CAD build for the part. Positions are in the model's coordinates, mm. Round coordinates to 2 decimals unless told otherwise and drop trailing zeros. Loops run counter-clockwise (first coordinate to the right, second up) from the corner with the lowest first, then second, coordinate; pieces in that order, holes last.
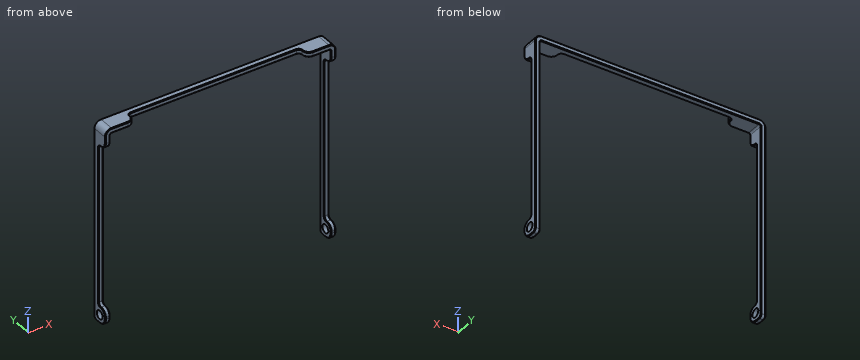
from build123d import *

# Parameters (mm, degrees)
EXTRUDE_1_DEPTH     = 5
FILLET_1_R          = 2
FILLET_2_R          = 0.5
FILLET_3_R          = 2.5
SKETCH_2_R          = 1.3
CUT_EXTRUDE_1_DEPTH = 100
SKETCH_3_W          = 52.2
SKETCH_3_H          = 6.2
CUT_EXTRUDE_2_DEPTH = 5
FILLET_5_R          = 1
SKETCH_4_W          = 49
SKETCH_4_H          = 8.82072143
CUT_EXTRUDE_3_DEPTH = 100
FILLET_6_R          = 1
FILLET_7_R          = 2
CHAMFER_1_SIZE      = 0.2


with BuildPart() as part:
    # 草图1 → 凸台-拉伸1 (new body)
    with BuildSketch(Plane(origin=(0, 0, 0), x_dir=(1, 0, 0), z_dir=(0, 1, 0))):
        Polygon((33.5, 29.25), (35, 29.25), (35, -30.75), (-35, -30.75), (-35, 29.25), (-33.5, 29.25), (-33.5, -29.25), (33.5, -29.25), align=None)
    extrude(amount=EXTRUDE_1_DEPTH)

    # 圆角1
    fillet_1_edges = [part.edges().sort_by_distance(p)[0] for p in [
        (35, 2.5, 30.75),
        (-35, 2.5, 30.75),
    ]]
    fillet(fillet_1_edges, radius=FILLET_1_R)

    # 圆角2
    fillet_2_edges = [part.edges().sort_by_distance(p)[0] for p in [
        (-33.5, 2.5, 29.25),
        (33.5, 2.5, 29.25),
    ]]
    fillet(fillet_2_edges, radius=FILLET_2_R)

    # 圆角3
    fillet_3_edges = [part.edges().sort_by_distance(p)[0] for p in [
        (-34.25, 0, -29.25),
        (34.25, 0, -29.25),
    ]]
    fillet(fillet_3_edges, radius=FILLET_3_R)

    # 草图2 → 切除-拉伸1 (cut)
    with BuildSketch(Plane.ZY.offset(35)):
        with Locations((-26.75, 2.5)):
            Circle(SKETCH_2_R)
    extrude(amount=-CUT_EXTRUDE_1_DEPTH, mode=Mode.SUBTRACT)

    # 草图3 → 切除-拉伸2 (cut)
    with BuildSketch(Plane.XY.offset(30.75)):
        Rectangle(SKETCH_3_W, SKETCH_3_H)
    extrude(amount=-CUT_EXTRUDE_2_DEPTH, mode=Mode.SUBTRACT)

    # 圆角5
    fillet_5_edges = [part.edges().sort_by_distance(p)[0] for p in [
        (-26.1, 3.1, 30),
        (26.1, 3.1, 30),
    ]]
    fillet(fillet_5_edges, radius=FILLET_5_R)

    # 草图4 → 切除-拉伸3 (cut)
    with BuildSketch(Plane.ZY.offset(35)):
        with Locations((0.25, -1.310360715)):
            Rectangle(SKETCH_4_W, SKETCH_4_H)
    extrude(amount=-CUT_EXTRUDE_3_DEPTH, mode=Mode.SUBTRACT)

    # 圆角6
    fillet_6_edges = [part.edges().sort_by_distance(p)[0] for p in [
        (34.25, 3.1, -24.25),
        (-34.25, 3.1, -24.25),
        (34.25, 3.1, 24.75),
        (-34.25, 3.1, 24.75),
        (-34.25, 5, -29.25),
        (34.25, 5, -29.25),
    ]]
    fillet(fillet_6_edges, radius=FILLET_6_R)

    # 圆角7
    fillet_7_edges = [part.edges().sort_by_distance(p)[0] for p in [
        (-34.25, 0, 24.75),
        (-34.25, 0, -24.25),
        (34.25, 0, -24.25),
        (34.25, 0, 24.75),
        (-26.1, 0, 30),
        (26.1, 0, 30),
    ]]
    fillet(fillet_7_edges, radius=FILLET_7_R)

    # 倒角1
    chamfer_1_edges = [part.edges().sort_by_distance(p)[0] for p in [
        (33.5, 5, 0.25),
        (-35, 5, 0.25),
        (-35, 2.05, -24.25),
        (-35, 3.1, 0.25),
        (-35, 3.25, -29.25),
        (-35, 4.707106781, -28.957106781),
        (-33.5, 3.25, -29.25),
        (-33.5, 3.1, 0.25),
        (-33.5, 2.05, -24.25),
        (-33.5, 4.707106781, -28.957106781),
        (33.5, 3.1, 0.25),
        (33.5, 2.05, 24.75),
        (33.5, 3.25, -29.25),
        (33.5, 4.707106781, -28.957106781),
        (35, 3.25, -29.25),
        (35, 3.1, 0.25),
        (35, 2.05, -24.25),
        (35, 4.707106781, -28.957106781),
        (33.5, 2.807106781, -23.957106781),
        (35, 2.807106781, -23.957106781),
        (33.5, 2.807106781, 24.457106781),
        (35, 2.807106781, 24.457106781),
        (-35, 2.807106781, 24.457106781),
        (-33.5, 2.807106781, 24.457106781),
        (-35, 2.807106781, -23.957106781),
        (-33.5, 2.807106781, -23.957106781),
        (35, 0, -26.5),
        (33.5, 2.05, -24.25),
        (33.5, 0, 27.75),
        (33.5, 0.585786438, 25.335786438),
        (33.5, 0.585786438, -24.835786438),
        (35, 2.05, 24.75),
        (35, 0.585786438, 25.335786438),
        (35, 0.585786438, -24.835786438),
        (-33.5, 0, -26.5),
        (-35, 2.05, 24.75),
        (-35, 0, 27.75),
        (-35, 0.585786438, 25.335786438),
        (-35, 0.585786438, -24.835786438),
        (-33.5, 2.05, 24.75),
        (-33.5, 0.585786438, 25.335786438),
        (-33.5, 0.585786438, -24.835786438),
        (-30.55, 0, 29.25),
        (26.1, 2.05, 30.75),
        (30.55, 0, 30.75),
        (26.685786438, 0.585786438, 30.75),
        (-26.685786438, 0.585786438, 30.75),
        (26.1, 2.05, 29.25),
        (26.685786438, 0.585786438, 29.25),
        (-26.685786438, 0.585786438, 29.25),
        (35, 0, 27.75),
        (35, 5, 0.25),
        (-30.55, 0, 30.75),
        (-34.414213562, 0, 30.164213562),
        (34.414213562, 0, 30.164213562),
        (0, 5, 30.75),
        (-34.414213562, 5, 30.164213562),
        (34.414213562, 5, 30.164213562),
        (30.55, 0, 29.25),
        (0, 5, 29.25),
        (-33.5, 0, 27.75),
        (-33.5, 5, 0.25),
        (33.353553391, 0, 29.103553391),
        (33.353553391, 5, 29.103553391),
        (-33.353553391, 0, 29.103553391),
        (-33.353553391, 5, 29.103553391),
        (33.5, 0, -26.5),
        (33.5, 0.732233047, -28.517766953),
        (-35, 0, -26.5),
        (35, 0.732233047, -28.517766953),
        (-35, 0.732233047, -28.517766953),
        (-33.5, 0.732233047, -28.517766953),
        (0, 3.1, 30.75),
        (0, 3.1, 29.25),
        (-26.1, 2.05, 30.75),
        (-26.1, 2.05, 29.25),
        (25.807106781, 2.807106781, 30.75),
        (25.807106781, 2.807106781, 29.25),
        (-25.807106781, 2.807106781, 30.75),
        (-25.807106781, 2.807106781, 29.25),
    ]]
    chamfer(chamfer_1_edges, length=CHAMFER_1_SIZE)


solid = part.part
Item 1: Flat gauge pins, fed straight in: P1, Ø2.5, axis at x = -3.5, y = 2, coming from the -Z side; P2, Ø0.9, axis at x = 34, z = -9.5, coming from the -Y side. Where does each tip first touch, or does it go through?
Verdict:
P1: stops at z = 29.3
P2: stops at y = 3.1
Item 2: Cut at C-C (x = 1.5). List the corners of the cut face in (y, z).
Verdict:
outline: (3.1, 29.45) - (3.3, 29.25) - (4.8, 29.25) - (5, 29.45) - (5, 30.55) - (4.8, 30.75) - (3.3, 30.75) - (3.1, 30.55) - close
Item 3: Cut at B-B (x = 29.5). List the corners of the cut face in (y, z), plus the area to 3 significant figures.
Verdict:
outline: (0, 29.45) - (0.2, 29.25) - (4.8, 29.25) - (5, 29.45) - (5, 30.55) - (4.8, 30.75) - (0.2, 30.75) - (0, 30.55) - close
area: 7.42 mm2
Item 4: Cut at A-A (z = 5.5). List the corners of the cut face in (x, y).
Verdict:
outline: (-35, 3.3) - (-34.8, 3.1) - (-33.7, 3.1) - (-33.5, 3.3) - (-33.5, 4.8) - (-33.7, 5) - (-34.8, 5) - (-35, 4.8) - close; (33.5, 3.3) - (33.7, 3.1) - (34.8, 3.1) - (35, 3.3) - (35, 4.8) - (34.8, 5) - (33.7, 5) - (33.5, 4.8) - close
Item 5: Wall check: L1, parallel to X at y = 4.75, z = 4; L2, parallel to Y at x = 33.95, z = -26.75; L3, parallel to Z at x = 27, y = 4.8. Give the ranges that are in metal, low to high.
Verdict:
L1: x = -35 to -33.5, 33.5 to 35
L2: y = 0 to 1.2, 3.8 to 5
L3: z = 29.25 to 30.75
